Can you work these out from the model? Positions are in its coordinate system, mm. Face numbers are marked on the shaded views. A direction names the side the tool comes from. Coordinates: 2 decimals unless noted, no trailing zeros. Loops run counter-clockwise (first coordinate to the right, second up) from the corner with the lowest first, then second, coordinate; pieces in that order, holes last. Notation, with made-up numbers: M -10,2.5 L 24,2.5 A35 ccw 24,37.5 Z; hole C 59,36 d11. An arc over 180 degrees is marked long. Return JSON: item names as keys, results as strings. Group by question number.
```python
from build123d import *

# Parameters (mm, degrees)
BOSS_EXTRUDE1_DEPTH = 6


with BuildPart() as part:
    # Sketch1 → Boss-Extrude1 (new body)
    with BuildSketch(Plane.XY):
        with BuildLine():
            Line((3, 6), (5, 8))
            Line((5, 8), (5, 19))
            ThreePointArc((5, 19), (5.292893219, 19.707106781), (6, 20))
            Line((6, 20), (49, 20))
            ThreePointArc((49, 20), (55, 26), (49, 32))
            Line((49, 32), (0, 32))
            ThreePointArc((0, 32), (-3.535533906, 30.535533906), (-5, 27))
            Line((-5, 27), (-5, 8))
            Line((-5, 8), (-3, 6))
            Line((-3, 6), (-3, 0))
            Line((-3, 0), (3, 0))
            Line((3, 0), (3, 6))
        make_face()
        with BuildLine():
            Line((0, 27), (49, 27))
            ThreePointArc((49, 27), (50, 26), (49, 25))
            Line((49, 25), (0, 25))
            ThreePointArc((0, 25), (-1, 26), (0, 27))
        make_face(mode=Mode.SUBTRACT)
    boss_extrude1 = extrude(amount=BOSS_EXTRUDE1_DEPTH)

    # Mirror1: Boss-Extrude1 across plane
    add(boss_extrude1.mirror(Plane(origin=(-3, 0, 6), x_dir=(0, 0, 1), z_dir=(0, 1, 0))))


solid = part.part
```
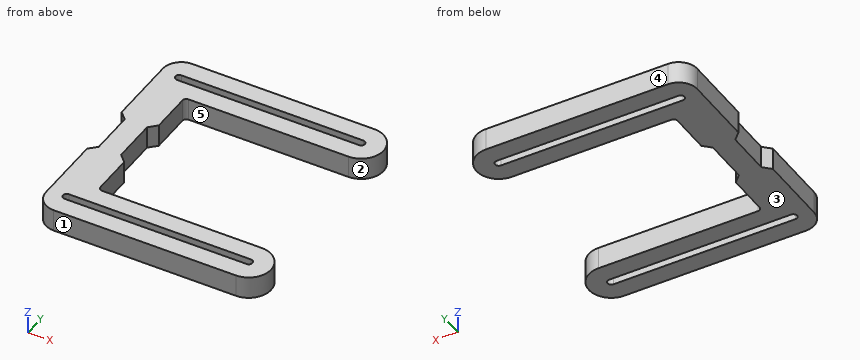
1) Suppose I cut it at B-B, the plane z = 2.9. List the corners of the cut face in (x, y) for me.
2) Suppose I cut it at C-C, the plane x = 31. List the corners of the cut face in (y, z) for me.
3) If we mould it in two halves opening along Y, with no side actions, what happens to the marked faces 1, 2 and 3? For each: +Y half, -Y half, draft (parallel to the pull), parting line (faces both ways), or undercut.
4) For pin 1 (1.8 mm diameter, centred on y = -14.5, z = 3, fed in from +X); pin 2 (1.8 mm diameter, centred on y = -2, z = 2.5, fed in from -X), each with a flat end and sliding along its axis, tell me the tip position at first contact or that it passes through.
5) For the marked faces 4 and 5, which set-ups out of +Z, -Z, +X, -X, +Y, -Y let a thin tool reach every point of the face, with its end or its side?
6) Suppose I cut it at A-A, the plane y = 26. List the corners of the cut face in (x, z) for me.
7) If I drill on line 1 (Y direction, x = 31.5, z = 3.25); line 2 (X direction, y = 16, z = 5.35); line 3 (Y direction, x = 5.5, z = 3.75), over which ranges is the centre line in solid material (lowest first)? Write a range as from..to.
8) Suppose I cut it at D-D, the plane y = 14. List the corners of the cut face in (x, z) for me.
Returned:
{
 "1": {"outline": "M -5,-27 A5 ccw 0,-32 L 49,-32 A6 ccw 49,-20 L 6,-20 A1 cw 5,-19 L 5,-8 L 3,-6 L 3,6 L 5,8 L 5,19 A1 cw 6,20 L 49,20 A6 ccw 49,32 L 0,32 A5 ccw -5,27 L -5,8 L -3,6 L -3,-6 L -5,-8 Z; hole M 0,-27 L 49,-27 A1 ccw 49,-25 L 0,-25 A1 ccw Z; hole M 0,25 L 49,25 A1 ccw 49,27 L 0,27 A1 ccw Z"},
 "2": {"outline": "M -32,0 L -27,0 L -27,6 L -32,6 Z; M -25,0 L -20,0 L -20,6 L -25,6 Z; M 20,0 L 25,0 L 25,6 L 20,6 Z; M 27,0 L 32,0 L 32,6 L 27,6 Z"},
 "3": {"face 1": "-Y half", "face 2": "undercut", "face 3": "draft"},
 "4": {"pin 1": "stops at x = 5", "pin 2": "stops at x = -3"},
 "5": {"face 4": "+Z, -Z, +X, -X, +Y", "face 5": "+Z, -Z, +X"},
 "6": {"outline": "M -5,0 L -1,0 L -1,6 L -5,6 Z; M 50,0 L 55,0 L 55,6 L 50,6 Z"},
 "7": {"line 1": "y = -32..-27, -25..-20, 20..25, 27..32", "line 2": "x = -5..5", "line 3": "y = -32..-27, -25..-19.87, 19.87..25, 27..32"},
 "8": {"outline": "M -5,0 L 5,0 L 5,6 L -5,6 Z"}
}
